Work out the finished part from the listing and answer in its coordinate system (mm). Coordinates: 2 decimals unless noted, no trailing zeros. Write each loop counter-clockwise with the first axis right and the second up, starting at its lowest first coordinate (ties: lowest second). Pieces come first, ordered by that corner, then holes. Notation, with made-up numbers: (-32.5, -2) - (13.5, -2) arc R31 ccw to (13.5, 25) - close; hole circle Ø8 at (-24.5, 77). An arc over 180 degrees is marked (long way). Use one line per item in the form item = value. Start each with the question number.
Item 1: A cutting plane is placed at A-A (z = 0). Write down the section's boundary in (x, y).
Item 2: A cutting plane is placed at B-B (y = 2.5). Write down the section's boundary in (x, z).
Item 3: A cutting plane is placed at C-C (z = 9). Write down the section's boundary in (x, y).
Item 4: Consider probe 1 along X at (y, z) = (1.65, 0); probe 2 along X at (y, z) = (0.5, 2); probe 3 along X at (y, z) = (0.9, -8). Determine where each line is inside the solid, lowest interval first.
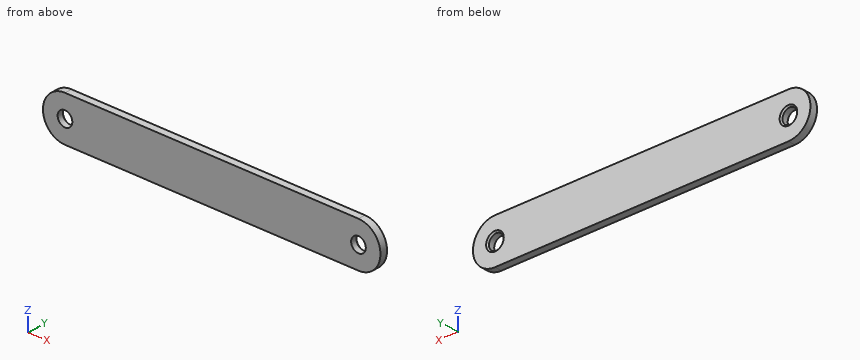
from build123d import *

# Parameters (mm, degrees)
SKETCH1_R           = 5
BOSS_EXTRUDE1_DEPTH = 5
CHAMFER1_SIZE       = 1
CHAMFER2_SIZE       = 1


with BuildPart() as part:
    # Sketch1 → Boss-Extrude1 (new body)
    with BuildSketch(Plane(origin=(0, 0, 0), x_dir=(1, 0, 0), z_dir=(0, 1, 0))):
        with BuildLine():
            Line((0, 15), (200, 15))
            ThreePointArc((200, 15), (215, 0), (200, -15))
            Line((200, -15), (0, -15))
            ThreePointArc((0, -15), (-15, 0), (0, 15))
        make_face()
        with Locations(Location((0, 0, 0), (0, 0, 270))):
            Circle(SKETCH1_R, mode=Mode.SUBTRACT)
        with Locations(Location((200, 0, 0), (0, 0, 270))):
            Circle(SKETCH1_R, mode=Mode.SUBTRACT)
    extrude(amount=BOSS_EXTRUDE1_DEPTH)

    # Chamfer1
    chamfer1_edges = [part.edges().sort_by_distance(p)[0] for p in [
        (200, 5, -5),
    ]]
    chamfer(chamfer1_edges, length=CHAMFER1_SIZE)

    # Chamfer2
    chamfer2_edges = [part.edges().sort_by_distance(p)[0] for p in [
        (0, 5, -5),
    ]]
    chamfer(chamfer2_edges, length=CHAMFER2_SIZE)


solid = part.part
Answer:
q1.outline = (-15, 0) - (-5, 0) - (-5, 4) - (-6, 5) - (-15, 5) - close; (5, 0) - (195, 0) - (195, 4) - (194, 5) - (6, 5) - (5, 4) - close; (205, 0) - (215, 0) - (215, 5) - (206, 5) - (205, 4) - close
q2.outline = (0, -15) - (200, -15) arc R15 ccw to (200, 15) - (0, 15) arc R15 ccw to start; hole circle Ø10 at (0, 0); hole circle Ø10 at (200, 0)
q3.outline = (-12, 0) - (212, 0) - (212, 5) - (-12, 5) - close
q4.probe_1 = -15 to -5, 5 to 195, 205 to 215
q4.probe_2 = -14.87 to -4.58, 4.58 to 195.42, 204.58 to 214.87
q4.probe_3 = -12.69 to 212.69
